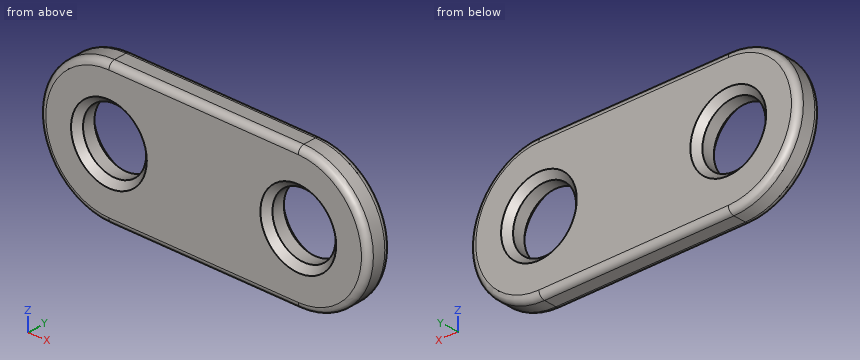
```python
from build123d import *

# Parameters (mm, degrees)
F0_R     = 2.5
F1_DEPTH = 2
F2_SIZE  = 0.5
F3_R     = 0.5


with BuildPart() as f1:
    # F0 (on Front) → F1 (new body)
    with BuildSketch(Plane.XZ):
        with BuildLine():
            Line((8.957038, 9.614641), (-6.042962, 9.614641))
            ThreePointArc((-6.042962, 9.614641), (-11.542962, 4.114641), (-6.042962, -1.385359))
            Line((-6.042962, -1.385359), (8.957038, -1.385359))
            ThreePointArc((8.957038, -1.385359), (14.457038, 4.114641), (8.957038, 9.614641))
        make_face()
        with Locations((-6.042962, 4.114641)):
            Circle(F0_R, mode=Mode.SUBTRACT)
        with Locations((8.957038, 4.114641)):
            Circle(F0_R, mode=Mode.SUBTRACT)
    extrude(amount=F1_DEPTH)

    # F2
    f2_edges = [f1.edges().sort_by_distance(p)[0] for p in [
        (-8.542962, -2, 4.114641),
        (6.457038, -2, 4.114641),
        (-8.542962, 0, 4.114641),
        (6.457038, 0, 4.114641),
    ]]
    chamfer(f2_edges, length=F2_SIZE)

    # F3
    f3_edges = [f1.edges().sort_by_distance(p)[0] for p in [
        (1.457038, -2, -1.385359),
        (1.457038, 0, -1.385359),
    ]]
    fillet(f3_edges, radius=F3_R)


solid = f1.part
```
Can you work these out from the model? Positions are in its coordinate system, mm. Coordinates: 2 decimals unless noted, no trailing zeros. Order: outer loops, then holes, each group sorted by start corner. A loop starts at its lowest first (then second) coordinate and runs counter-clockwise, first axis right, second up. Notation, with made-up numbers: (81.25, 81.5) -> (104.25, 81.5) arc R21 cw to (104.25, 100.5) -> close; hole circle Ø3 at (58, -2). An arc over 180 degrees is marked (long way). Write each question's results on one line, items separated by ' | '.
Item 1: I want a section at B-B, the plane z = 4.5. Count the separate pieces of the cut face and the enclosed holes in it, then the cut area to 3 significant figures.
Results are:
separate pieces: 3 | enclosed holes: 0 | area: 31.0 mm²
Item 2: I'm going to push a flat-ended pin straight in: pin 1 Ø4.5 at (x, z) = (-6.04, 4.11) entering from +Y. Where does the tip first touch, or does it pass through?
Results are:
pin 1: through
Item 3: If I drill on line 1 along X through (y, z) = (-1.4, 5); line 2 along X through (y, z) = (-1.35, 2.5); line 3 along Z through (x, y) = (-8.25, -1.7), over which ranges is the centre line in solid material (lowest first)?
Results are:
line 1: -11.47 to -8.38, -3.7 to 6.62, 11.3 to 14.39 | line 2: -11.3 to -7.95, -4.13 to 7.05, 10.87 to 14.21 | line 3: -0.88 to 2.56, 5.67 to 9.11
Item 4: I want a section at A-A, the plane y = -1.1. Write out the boundary of the cut face in (x, z).
Results are:
outline: (-6.04, -1.39) -> (8.96, -1.39) arc R5.5 ccw to (8.96, 9.61) -> (-6.04, 9.61) arc R5.5 ccw to start; hole circle Ø5 at (-6.04, 4.11); hole circle Ø5 at (8.96, 4.11)
